Part model, mm, in its own coordinate system. Face numbers are marked on the shaded views. A direction names the side the tool comes from. Coordinates: 2 decimals unless noted, no trailing zeros. Loops run counter-clockwise (first coordinate to the right, second up) from the corner with the lowest first, then second, coordinate; pieces in that order, holes last. Notation, with made-up numbers: (83, 17) - (131, 17) arc R28 cw to (131, 40) - close; hole circle Ø2 at (-4.75, 85). An arc over 180 degrees is marked (long way). One line per question, with ' | ' between items. Start each with the question number.
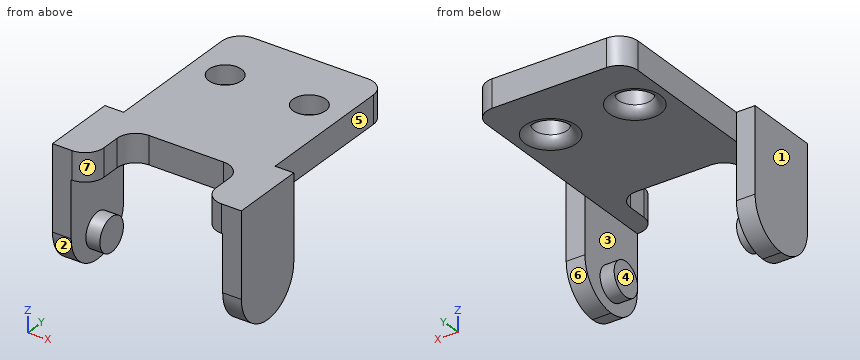
from build123d import *

# Parameters (mm, degrees)
ESQUISSE1_W             = 16.2
ESQUISSE1_H             = 25
BOSS_EXTRU_1_DEPTH      = 3
ESQUISSE2_W             = 13
ESQUISSE2_H             = 8
BOSS_EXTRU_2_DEPTH      = 2
ESQUISSE3_R             = 1.8
BOSS_EXTRU_3_DEPTH      = 1.5
ESQUISSE5_W             = 13
ESQUISSE5_H             = 8
BOSS_EXTRU_4_DEPTH      = 2
ESQUISSE6_R             = 1.8
BOSS_EXTRU_5_DEPTH      = 1.5
ENL_V_MAT_EXTRU_1_REACH = 34.5
ESQUISSE7_W             = 12
ESQUISSE7_H             = 6
ENL_V_MAT_EXTRU_2_REACH = 34.5
ESQUISSE8_R             = 1.75
CONG_1_R                = 1
CONG_2_R                = 4
CONG_3_R                = 2
CONG_4_R                = 2


with BuildPart() as part:
    # Esquisse1 → Boss.-Extru.1 (new body)
    with BuildSketch(Plane.XY):
        with Locations((8.1, 12.5)):
            Rectangle(ESQUISSE1_W, ESQUISSE1_H)
    extrude(amount=BOSS_EXTRU_1_DEPTH)

    # Esquisse2 → Boss.-Extru.2 (add)
    with BuildSketch(Plane.ZY):
        with Locations((-3.5, 4)):
            Rectangle(ESQUISSE2_W, ESQUISSE2_H)
    extrude(amount=BOSS_EXTRU_2_DEPTH)

    # Esquisse3 → Boss.-Extru.3 (add)
    with BuildSketch(Plane(origin=(0, 0, 0), x_dir=(0, 0, -1), z_dir=(1, 0, 0))):
        with Locations(Location((7, 4.035774971, 0), (0, 0, 180))):
            Circle(ESQUISSE3_R)
    extrude(amount=BOSS_EXTRU_3_DEPTH)

    # Esquisse5 → Boss.-Extru.4 (add)
    with BuildSketch(Plane(origin=(16.2, 0, 0), x_dir=(0, 0, -1), z_dir=(1, 0, 0))):
        with Locations((3.5, 4)):
            Rectangle(ESQUISSE5_W, ESQUISSE5_H)
    extrude(amount=BOSS_EXTRU_4_DEPTH)

    # Esquisse6 → Boss.-Extru.5 (add)
    with BuildSketch(Plane.ZY.offset(-16.2)):
        with Locations((-7, 3.879731229)):
            Circle(ESQUISSE6_R)
    extrude(amount=BOSS_EXTRU_5_DEPTH)

    # Esquisse7 → Enlèv. mat.-Extru.1 (cut, up to next)
    with BuildSketch(Plane(origin=(0, 0, 0), x_dir=(-1, 0, 0), z_dir=(0, 0, -1)), mode=Mode.PRIVATE) as enl_v_mat_extru_1_sk1:
        with Locations((-8.1, 3)):
            Rectangle(ESQUISSE7_W, ESQUISSE7_H)
    enl_v_mat_extru_1_tool1 = extrude(enl_v_mat_extru_1_sk1.sketch, amount=-ENL_V_MAT_EXTRU_1_REACH, mode=Mode.PRIVATE) & part.part
    add(enl_v_mat_extru_1_tool1.solids().sort_by_distance((8.1, 3, 0))[0], mode=Mode.SUBTRACT)

    # Esquisse8 → Enlèv. mat.-Extru.2 (cut, up to next)
    with BuildSketch(Plane(origin=(0, 0, 0), x_dir=(-1, 0, 0), z_dir=(0, 0, -1)), mode=Mode.PRIVATE) as enl_v_mat_extru_2_sk1:
        with Locations((-12.6, 18.360124913)):
            Circle(ESQUISSE8_R)
    enl_v_mat_extru_2_tool1 = extrude(enl_v_mat_extru_2_sk1.sketch, amount=-ENL_V_MAT_EXTRU_2_REACH, mode=Mode.PRIVATE) & part.part
    # Esquisse8 → Enlèv. mat.-Extru.2 (cut, up to next)
    with BuildSketch(Plane(origin=(0, 0, 0), x_dir=(-1, 0, 0), z_dir=(0, 0, -1)), mode=Mode.PRIVATE) as enl_v_mat_extru_2_sk2:
        with Locations((-3.6, 18.360124913)):
            Circle(ESQUISSE8_R)
    enl_v_mat_extru_2_tool2 = extrude(enl_v_mat_extru_2_sk2.sketch, amount=-ENL_V_MAT_EXTRU_2_REACH, mode=Mode.PRIVATE) & part.part
    add(enl_v_mat_extru_2_tool1.solids().sort_by_distance((12.6, 18.360125, 0))[0], mode=Mode.SUBTRACT)
    add(enl_v_mat_extru_2_tool2.solids().sort_by_distance((3.6, 18.360125, 0))[0], mode=Mode.SUBTRACT)

    # Congé1
    cong_1_edges = [part.edges().sort_by_distance(p)[0] for p in [
        (14.35, 18.360124913, 0),
        (5.35, 18.360124913, 0),
    ]]
    fillet(cong_1_edges, radius=CONG_1_R)

    # Congé2
    cong_2_edges = [part.edges().sort_by_distance(p)[0] for p in [
        (-1, 8, -10),
        (-1, 0, -10),
        (17.2, 0, -10),
        (17.2, 8, -10),
    ]]
    fillet(cong_2_edges, radius=CONG_2_R - 0.0001)  # a hair under: the kernel refuses the full size

    # Congé3
    cong_3_edges = [part.edges().sort_by_distance(p)[0] for p in [
        (14.1, 0, 1.5),
        (14.1, 6, 1.5),
        (2.1, 6, 1.5),
        (2.1, 0, 1.5),
    ]]
    fillet(cong_3_edges, radius=CONG_3_R)

    # Congé4
    cong_4_edges = [part.edges().sort_by_distance(p)[0] for p in [
        (0, 25, 1.5),
        (16.2, 25, 1.5),
    ]]
    fillet(cong_4_edges, radius=CONG_4_R)


solid = part.part
1) Band-saw the part on D-D on z = 1.75. List the corners of the cut face in (x, y).
2) Tool access for the marked faces 4, 5, 6 and 7: list every direction of +Z, -Z, +X, -X, +Y, -Y with a clear straight run to the whole face (end or side of a thin tool).
3) Wall check: line 1 along X through (y, z) = (3.75, -4.25); line 2 along Y through (x, z) = (8.5, 1.75); line 3 along Z through (x, y) = (15.25, 9). Give the ranges that are in metal, low to high. Write a range as [from, to].
4) Band-saw the part on C-C on y = 4.75. List the corners of the cut face in (x, z).
5) Pin check, flat tips, straight feed: pin 1 Ø1.5 at (x, z) = (11, -1) entering from +Y; pin 2 Ø4 at (x, y) = (3.6, 18.36) entering from -Z; pin 3 Ø4.5 at (x, y) = (12.6, 18.36) entering from -Z; pin 4 Ø1.5 at (y, z) = (18, 2) entering from +X. Stop position of each tip, or through.
6) Band-saw the part on B-B on x = 12.6. List the corners of the cut face in (y, z).
7) Band-saw the part on A-A on z = -2.5. List the corners of the cut face in (x, y), then the cut area to 3 significant figures.
8) Mould opens along X. For the marked faces 1, 2 and 3 say: +X half, -X half, draft (parallel to the pull), parting line (faces both ways), or undercut.
Values found:
1) outline: (-2, 0) - (0.1, 0) arc R2 ccw to (2.1, 2) - (2.1, 4) arc R2 cw to (4.1, 6) - (12.1, 6) arc R2 cw to (14.1, 4) - (14.1, 2) arc R2 ccw to (16.1, 0) - (18.2, 0) - (18.2, 8) - (16.2, 8) - (16.2, 23) arc R2 ccw to (14.2, 25) - (2, 25) arc R2 ccw to (0, 23) - (0, 8) - (-2, 8) - close; hole circle Ø3.5 at (3.6, 18.36); hole circle Ø3.5 at (12.6, 18.36)
2) face 4: -Z, +Y, -Y | face 5: +Z, -Z, +X, +Y | face 6: -Z, +X, -X, +Y | face 7: +Z, -Z, -Y
3) line 1: [-2, 0], [16.2, 18.2] | line 2: [6, 25] | line 3: [0, 3]
4) outline: (-2, -9.93) - (0, -9.93) - (0, -8.65) - (1.5, -8.65) - (1.5, -5.35) - (0, -5.35) - (0, 0) - (2.25, 0) - (2.25, 3) - (-2, 3) - close; (13.95, 0) - (16.2, 0) - (16.2, -5.42) - (14.7, -5.42) - (14.7, -8.58) - (16.2, -8.58) - (16.2, -9.93) - (18.2, -9.93) - (18.2, 3) - (13.95, 3) - close
5) pin 1: through | pin 2: z = 0.34 | pin 3: z = 0.13 | pin 4: x = 16.2
6) outline: (5.94, 0) - (15.61, 0) arc R1 ccw to (16.61, 1) - (16.61, 3) - (5.94, 3) - close; (20.11, 1) arc R1 ccw to (21.11, 0) - (25, 0) - (25, 3) - (20.11, 3) - close
7) outline: (-2, 0) - (0, 0) - (0, 8) - (-2, 8) - close; (16.2, 0) - (18.2, 0) - (18.2, 8) - (16.2, 8) - close | area: 32.0 mm²
8) face 1: -X half | face 2: draft | face 3: undercut
